```python
from build123d import *

# Parameters (mm, degrees)
SKETCH1_W                                      = 110
SKETCH1_H                                      = 23
BOSS_EXTRUDE1_DEPTH                            = 15
F_6_0_6_DIAMETER_HOLE1_D                       = 6
F_6_0_6_DIAMETER_HOLE1_DEPTH                   = 6.01
F_6_0_6_DIAMETER_HOLE1_TIP                     = 1.802581857
CSK_FOR_M3_5_FLAT_HEAD_MACHINE_SCREW1_AT_COUNT = 2
CSK_FOR_M3_5_FLAT_HEAD_MACHINE_SCREW1_AT_PITCH = 100
CUT_EXTRUDE1_DEPTH                             = 62.473571557


with BuildPart() as part:
    # Sketch1 → Boss-Extrude1 (new body)
    with BuildSketch(Plane(origin=(-7.5, 0, 0), x_dir=(0, -1, 0), z_dir=(-1, 0, 0))):
        with Locations((0, -11.5)):
            Rectangle(SKETCH1_W, SKETCH1_H)
    extrude(amount=-BOSS_EXTRUDE1_DEPTH)

    # Ø6.0 (6) Diameter Hole1
    with Locations(Plane.XY):
        with Locations((0, 30), (0, -30)):
            Hole(F_6_0_6_DIAMETER_HOLE1_D / 2, depth=F_6_0_6_DIAMETER_HOLE1_DEPTH)
            with Locations((0, 0, -(F_6_0_6_DIAMETER_HOLE1_DEPTH + F_6_0_6_DIAMETER_HOLE1_TIP / 2))):  # 118° drill point
                Cone(0, F_6_0_6_DIAMETER_HOLE1_D / 2, F_6_0_6_DIAMETER_HOLE1_TIP, mode=Mode.SUBTRACT)

    # Sketch4 → CSK for M3.5 Flat Head Machine Screw1 (revolve, cut)
    with BuildSketch(Plane(origin=(0, 50, 0), x_dir=(0, -1, 0), z_dir=(1, 0, 0))):
        Polygon((0, 0), (0, 23), (2.1, 23), (2.1, 6.540774559), (3, 6), (3, 0), align=None)
    csk_for_m3_5_flat_head_machine_screw1 = revolve(axis=Axis((0, 50, 6.35), (0, 0, -1)), mode=Mode.SUBTRACT)

    # CSK for M3.5 Flat Head Machine Screw1 at: CSK for M3.5 Flat Head Machine Screw1 ×2
    with Locations(*[(0, -i * CSK_FOR_M3_5_FLAT_HEAD_MACHINE_SCREW1_AT_PITCH, 0) for i in range(1, CSK_FOR_M3_5_FLAT_HEAD_MACHINE_SCREW1_AT_COUNT)]):
        add(csk_for_m3_5_flat_head_machine_screw1, mode=Mode.SUBTRACT)

    # Sketch6 → Cut-Extrude1 (cut, through all)
    with BuildSketch(Plane(origin=(7.5, 0, 0), x_dir=(0, 0, -1), z_dir=(1, 0, 0))):
        Polygon((23, -55), (22.040044543, 55), (23, 55), align=None)
    extrude(amount=-CUT_EXTRUDE1_DEPTH, mode=Mode.SUBTRACT)


solid = part.part
```
Here's how the part is built. I have some questions about the finished solid (model axes, mm). A direction names the side the tool comes from. Coordinates: 2 decimals unless noted, no trailing zeros. Order: outer loops, then holes, each group sorted by start corner. A loop starts at its lowest first (then second) coordinate and runs counter-clockwise, first axis right, second up.
Item 1: If we section it at C-C, the plane x = -5.5: List the corners of the cut face in (y, z) for me, then the cut area to 3 significant figures.
Response values:
outline: (-55, -23) - (55, -22.04) - (55, 0) - (-55, 0) - close
area: 2,480 mm2
Item 2: I need wall thicknesses on probe 1 along Y at (x, z) = (0, -1.75); probe 2 along Y at (x, z) = (0, -11); probe 3 along X at (y, z) = (50, -2.9). Which ranges of each line are inside material? Lowest first, please.
Response values:
probe 1: y = -55 to -53, -47 to -33, -27 to 27, 33 to 47, 53 to 55
probe 2: y = -55 to -52.1, -47.9 to 47.9, 52.1 to 55
probe 3: x = -7.5 to -3, 3 to 7.5
Item 3: Thinking about a two-plate mould opening in X: for faces 3 (the face through (0, 55, -11)), 4 (the face through (2.21, 32.03, -3.05)), 5 (the face through (0, -47, -3)), 6 (the face through (7.5, 1, -11)), which applies, pulls with the +X half, pulls with the -X half, needs draft (parallel to the pull), parting line crosses it, or undercut?
Response values:
face 3: needs draft
face 4: undercut
face 5: undercut
face 6: pulls with the +X half
Item 4: If we section it at B-B, the plane y = 50: List the corners of the cut face in (x, z) for me.
Response values:
outline: (-7.5, -22.08) - (-2.1, -22.08) - (-2.1, -6.54) - (-3, -6) - (-3, 0) - (-7.5, 0) - close; (2.1, -22.08) - (7.5, -22.08) - (7.5, 0) - (3, 0) - (3, -6) - (2.1, -6.54) - close
Item 5: If we section it at D-D, the plane y = -7.5: List the corners of the cut face in (x, z) for me.
Response values:
outline: (-7.5, -22.59) - (7.5, -22.59) - (7.5, 0) - (-7.5, 0) - close
Item 6: If we section it at A-A, the plane z = -19: List the corners of the cut face in (x, y) for me, then the cut area to 3 significant figures.
Response values:
outline: (-7.5, -55) - (7.5, -55) - (7.5, 55) - (-7.5, 55) - close; hole circle Ø4.2 at (0, -50); hole circle Ø4.2 at (0, 50)
area: 1,620 mm2
Item 7: Which directions (+Z, -Z, +X, -X, +Y, -Y) give clear straight access to the entire face, cutting with the end or side of a thin tool? Please do faces 1 (the face through (0, 1, 0)), 2 (the face through (0.65, -32.93, -3.05)).
Response values:
face 1: +Z, +X, -X, +Y, -Y
face 2: +Z
Item 8: I'm going to push flat-ended pins straight in: pin 1 Ø8 at (x, y) = (5, -18) entering from -Z; pin 2 Ø6.5 at (x, y) = (0, 50) entering from -Z; pin 3 Ø2 at (x, y) = (-5, -10) entering from -Z; pin 4 Ø3.5 at (x, y) = (0, -50) entering from +Z. Where does each tip first touch, or does it pass through?
Response values:
pin 1: stops at z = -22.71
pin 2: stops at z = -22.11
pin 3: stops at z = -22.62
pin 4: passes through
